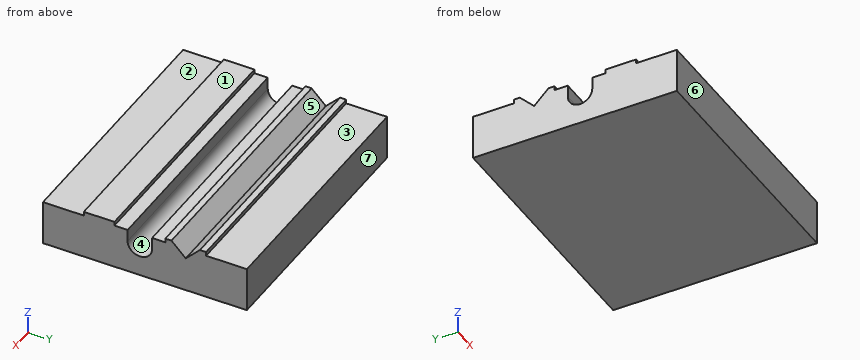
```python
from build123d import *

# Parameters (mm, degrees)
F1_DEPTH = 125


with BuildPart() as f1:
    # F0 (on Right) → F1 (new body)
    with BuildSketch(Plane.YZ):
        with BuildLine():
            Line((50, -11), (50, 11))
            Line((50, 11), (30, 11))
            Line((30, 11), (30, 13))
            Line((30, 13), (27, 13))
            Line((27, 13), (20, 6))
            Line((20, 6), (13, 13))
            Line((13, 13), (10, 13))
            Line((10, 13), (10, 11))
            Line((10, 11), (3.5, 11))
            Line((3.5, 11), (3.5, 5))
            ThreePointArc((3.5, 5), (-2.5, -1), (-8.5, 5))
            Line((-8.5, 5), (-8.5, 11))
            Line((-8.5, 11), (-15, 11))
            Line((-15, 11), (-15, 13))
            Line((-15, 13), (-30, 13))
            Line((-30, 13), (-30, 11))
            Line((-30, 11), (-50, 11))
            Line((-50, 11), (-50, -11))
            Line((-50, -11), (50, -11))
        make_face()
    extrude(amount=F1_DEPTH)


solid = f1.part
```
Read the model definition and answer for the solid it produces. Units are mm, in the model's axes. Face numbers are marked on the shaded views. A direction names the side the tool comes from. Round coordinates to 2 decimals unless told otherwise and drop trailing zeros. Write each loop counter-clockwise with the first axis right and the second up, starting at its lowest first coordinate (ties: lowest second). Pieces come first, ordered by that corner, then holes. Notation, with made-up numbers: (-6, 30.25) - (23, 30.25) arc R20 cw to (23, 60.25) - close; hole circle Ø4 at (42.5, 56.5). An arc over 180 degrees is marked (long way). One line per item, written item: value.
Q1. Find section C-C (y = -2.5). Determine the outline of the cut face in (x, z).
The answers:
outline: (0, -11) - (125, -11) - (125, -1) - (0, -1) - close
Q2. Each of these flat-tipped pins is pushed along its axis until it touches: P1, Ø6, axis at x = 83, y = -38.5, coming from the +Z side; P2, Ø2, axis at x = 93.5, z = 12.5, coming from the -Y side. Where does it stop, or does it pass through?
The answers:
P1: stops at z = 11
P2: stops at y = -30
Q3. Find section B-B (z = 3.25). Determine the outline of the cut face in (x, y), and give its area (3 significant figures).
The answers:
outline: (0, -50) - (125, -50) - (125, -8.24) - (0, -8.24) - close; (0, 3.24) - (125, 3.24) - (125, 50) - (0, 50) - close
area: 11,100 mm2
Q4. Find section A-A (x = 27). Determine the outline of the cut face in (y, z).
The answers:
outline: (-50, -11) - (50, -11) - (50, 11) - (30, 11) - (30, 13) - (27, 13) - (20, 6) - (13, 13) - (10, 13) - (10, 11) - (3.5, 11) - (3.5, 5) arc R6 cw to (-8.5, 5) - (-8.5, 11) - (-15, 11) - (-15, 13) - (-30, 13) - (-30, 11) - (-50, 11) - close
Q5. Find section D-D (y = 33). Determine the outline of the cut face in (x, z).
The answers:
outline: (0, -11) - (125, -11) - (125, 11) - (0, 11) - close
Q6. Which of the six approach directions +Z, -Z, +X, -X, +Y, -Y give full straight-line access (tool end or side, diameter ignored) to the marked faces 1, 2 and 3?
The answers:
face 1: +Z, +X, -X, +Y, -Y
face 2: +Z, +X, -X, -Y
face 3: +Z, +X, -X, +Y
Q7. For a pull along Y with two mould halves and no side action, classify the marked faces 4, 5, 6 and 7 as pulls with the +Y half, pulls with the -Y half, needs draft (parallel to the pull), parting line crosses it, or undercut.
The answers:
face 4: undercut
face 5: undercut
face 6: pulls with the -Y half
face 7: pulls with the +Y half
Q8. Straight lines are drawn through the part: line 1 (Y direction, x = 14, z = 8); line 2 (Y direction, x = 26, z = 10.75); line 3 (Y direction, x = 117, z = 5.5). For each, find the intervals that lie inside material, in ascending order. Write a range as from..to.
The answers:
line 1: y = -50..-8.5, 3.5..18, 22..50
line 2: y = -50..-8.5, 3.5..15.25, 24.75..50
line 3: y = -50..-8.5, 3.5..50
